Can you work these out from the drawing? Everything is in mm from the part's minimum corner. A direction names the side the tool comes from. Round coordinates to 2 decimals unless told otherwise and drop trailing zeros. Order: outer loops, then holes, each group sorted by start corner. A loop starts at its lowest first (then second) coordinate and runs counter-clockwise, first axis right, second up. Notation, with made-up numbers: (15.5, 2.25) - (33.5, 2.25) arc R19 cw to (33.5, 34.25) - close; hole circle Ø1 at (-30, 48). An arc over 180 degrees is marked (long way). Answer as a JSON object with one key per item and string values.
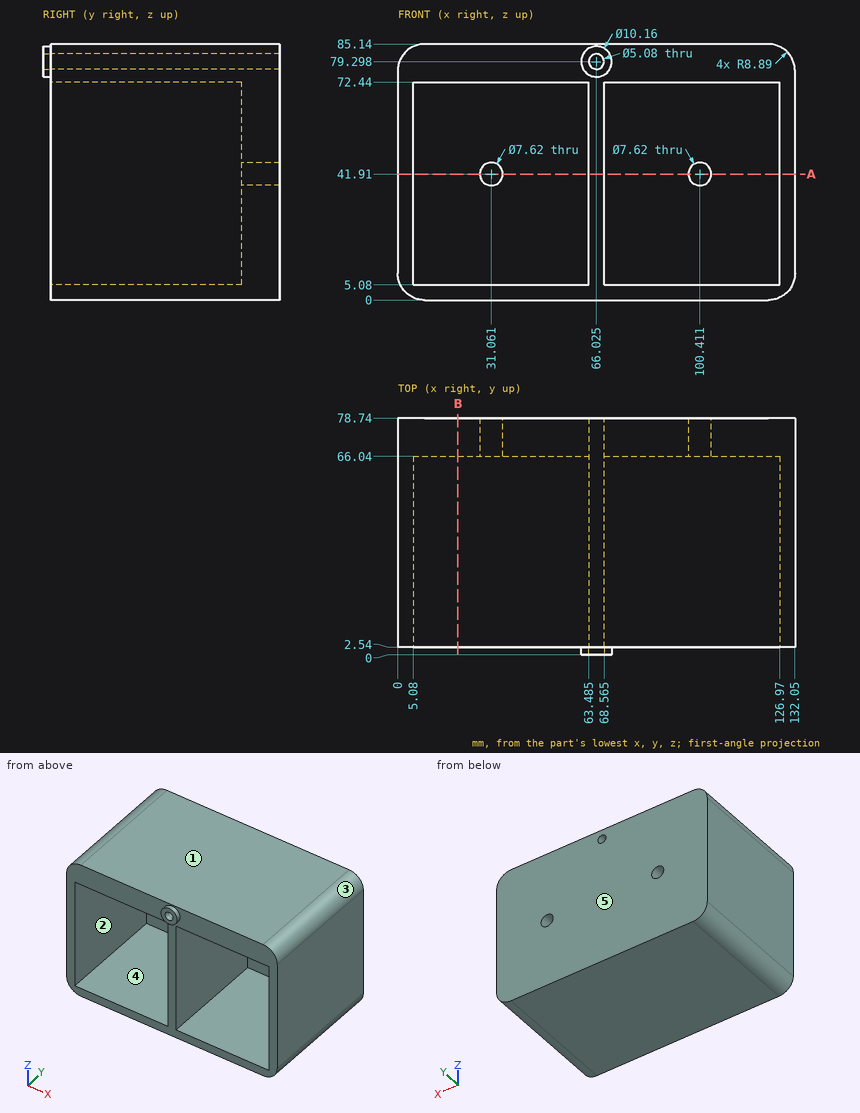
1. For the marked faces 1 and 2, which set-ups out of +Z, -Z, +X, -X, +Y, -Y let a thin tool reach every point of the face, with its end or its side?
Responses:
{"face 1": "+Z, +X, -X, +Y, -Y", "face 2": "-Y"}
2. Thinking about a two-plate mould opening in X: for the marked faces 3, 4 and 5, which applies, pulls with the +X half, pulls with the -X half, needs draft (parallel to the pull), parting line crosses it, or undercut?
Responses:
{"face 3": "pulls with the +X half", "face 4": "undercut", "face 5": "needs draft"}
3. Imagine slicing it at A-A (z = 41.91). Give the number of separate pieces and of enclosed holes in the cut face, plus the area to 3 significant figures.
Responses:
{"separate pieces": "3", "enclosed holes": "0", "area": "2,450 mm2"}
4. Imagine slicing it at B-B (x = 20). List the corners of the cut face in (y, z) for me, plus the area to 3 significant figures.
Responses:
{"outline": "(2.54, 0) - (78.74, 0) - (78.74, 85.14) - (2.54, 85.14) - (2.54, 72.44) - (66.04, 72.44) - (66.04, 5.08) - (2.54, 5.08) - close", "area": "2,210 mm2"}
5. If I drill on L1, parallel to Z at x = 96.5, y = 41.5; L2, parallel to X at y = 70, z = 41; L3, parallel to Y at x = 33.5, z = 20.5, over which ranges is the centre line in solid material (lowest first)? Write a range as [from, to].
Responses:
{"L1": "[0, 5.08], [72.44, 85.14]", "L2": "[0, 27.36], [34.76, 96.71], [104.11, 132.05]", "L3": "[66.04, 78.74]"}
6. For P1, Ø3, axis at x = 29.5, z = 67, coming from the -Y side, with a flat end and sliding along its axis, tell me the tip position at first contact or that it passes through.
Responses:
{"P1": "y = 66.04"}
